Design review of the part built by this model. Coordinates are the model's own, in mm. A direction names the side the tool comes from. Round coordinates to 2 decimals unless told otherwise and drop trailing zeros. Loops run counter-clockwise (first coordinate to the right, second up) from the corner with the lowest first, then second, coordinate; pieces in that order, holes last. Notation, with made-up numbers: M 16.5,20 L 29.5,20 A24 ccw 29.5,59 Z; hole C 89,54.5 d6. An arc over 180 degrees is marked long. One line per item, written item: value. Start each with the question number.
Item 1: We need section B-B (y = 43). Write out the cut boundary in (x, z), then the cut area to 3 significant figures.
Item 2: We need section C-C (y = 37). Write out the cut boundary in (x, z), then the cut area to 3 significant figures.
Item 3: Mouldability with a two-part tool opening along Y and no side actions: class faces 1 (the flat face through (32, 50, -9)), 2 (the cylindrical face through (57.16, 41.67, -11.66)), 3 (the flat face through (32, 3, -50)), 4 (the flat face through (32, 0, -25)) as released by +Y, released by -Y, zero draft, split by the parting line, or undercut.
Item 4: Clearance check with flat-ended pins moving along their axes: pin 1 (4 mm diameter, centred on x = 52, z = -22, fed in from -Y); pin 2 (12 mm diameter, centred on x = 20, z = -41.5, fed in from +Y); pin 3 (15.5 mm diameter, centred on x = 10.5, y = 41.5, fed in from -Z); pin 4 (6 mm diameter, centred on x = 49.5, y = 25.5, fed in from -Z). State where each tip first meets the part, or that it passes through.
Item 5: We need section A-A (x = 58). Write out the cut boundary in (y, z), then the cut area to 3 significant figures.
Item 6: For line 1 along Y through (x, z) = (7.5, -22.5); line 2 along Y through (x, z) = (10, -11); line 3 along Y through (x, z) = (4.5, -42), list the stretches that pass through material, from the lowest coordinate up.
Item 7: We need section D-D (x = 47.5). Write out the cut boundary in (y, z), then the cut area to 3 significant figures.
Item 8: For faces 5 (the flat face through (58, 41, -23)), 6 (the cylindrical face through (32.829, 42.902, -10.503)), 7 (the flat face through (25, 36, -11)), list the 3-axis set-ups (+Z, -Z, +X, -X, +Y, -Y) from which the entire face can be reached by the end or side of a thin tool; tool diameter is ignored.
from build123d import *

# Parameters (mm, degrees)
SKETCH1_W           = 65
SKETCH1_H           = 50
BOSS_EXTRUDE1_DEPTH = 6
SKETCH2_W           = 65
SKETCH2_H           = 10
BOSS_EXTRUDE2_DEPTH = 30
BOSS_EXTRUDE3_DEPTH = 14
SKETCH4_R           = 1.5
CUT_EXTRUDE1_DEPTH  = 23


with BuildPart() as part:
    # Sketch1 → Boss-Extrude1 (new body)
    with BuildSketch(Plane(origin=(0, 0, 0), x_dir=(1, 0, 0), z_dir=(0, 1, 0))):
        with Locations((32.5, 25)):
            Rectangle(SKETCH1_W, SKETCH1_H)
    extrude(amount=BOSS_EXTRUDE1_DEPTH)

    # Sketch2 → Boss-Extrude2 (add)
    with BuildSketch(Plane(origin=(0, 6, 0), x_dir=(1, 0, 0), z_dir=(0, 1, 0))):
        with Locations((32.5, 5)):
            Rectangle(SKETCH2_W, SKETCH2_H)
    extrude(amount=BOSS_EXTRUDE2_DEPTH)

    # Sketch3 → Boss-Extrude3 (add)
    with BuildSketch(Plane(origin=(0, 36, 0), x_dir=(1, 0, 0), z_dir=(0, 1, 0))):
        with BuildLine():
            Line((0, 0), (65, 0))
            Line((65, 0), (65, 23))
            Line((65, 23), (50.700274723, 23))
            ThreePointArc((50.700274723, 23), (32.5, 10.5), (14.299725277, 23))
            Line((14.299725277, 23), (0, 23))
            Line((0, 23), (0, 0))
        make_face()
    extrude(amount=BOSS_EXTRUDE3_DEPTH)

    # Sketch4 → Cut-Extrude1 (cut)
    with BuildSketch(Plane(origin=(0, 0, -23), x_dir=(-1, 0, 0), z_dir=(0, 0, -1))):
        with Locations((-57.850137362, 43)):
            Circle(SKETCH4_R)
        with Locations((-7.149862638, 43)):
            Circle(SKETCH4_R)
    extrude(amount=-CUT_EXTRUDE1_DEPTH, mode=Mode.SUBTRACT)


solid = part.part
A:
1. outline: M 0,-23 L 5.65,-23 L 5.65,0 L 0,0 Z; M 8.65,-23 L 14.3,-23 A19.5 cw 50.7,-23 L 56.35,-23 L 56.35,0 L 8.65,0 Z; M 59.35,-23 L 65,-23 L 65,0 L 59.35,0 Z
1. area: 1,030 mm2
2. outline: M 0,-23 L 14.3,-23 A19.5 cw 50.7,-23 L 65,-23 L 65,0 L 0,0 Z
2. area: 1,160 mm2
3. face 1: released by +Y
3. face 2: undercut
3. face 3: zero draft
3. face 4: released by -Y
4. pin 1: y = 0
4. pin 2: y = 6
4. pin 3: z = -23
4. pin 4: z = -10
5. outline: M 0,-50 L 6,-50 L 6,-10 L 36,-10 L 36,-23 L 41.51,-23 L 41.51,0 L 0,0 Z; M 44.49,-23 L 50,-23 L 50,0 L 44.49,0 Z
5. area: 853 mm2
6. line 1: 0 to 6, 36 to 41.54, 44.46 to 50
6. line 2: 0 to 6, 36 to 50
6. line 3: 0 to 6
7. outline: M 0,-50 L 6,-50 L 6,-10 L 36,-10 L 36,-17.54 L 50,-17.54 L 50,0 L 0,0 Z
7. area: 846 mm2
8. face 5: -Z, +X, -X, +Y
8. face 6: -Z, +Y
8. face 7: -Z, +X, -X
